Study the drawing (mm; zero at the part's minimum x, y, z) and answer. A direction names the side the tool comes from. Give positions to 0.01 mm unless a question says otherwise; leave off trailing zeros. Write each loop counter-clockwise with the first axis right and the second up, starting at its lowest first coordinate (ties: lowest second). Pieces come first, ordered by that corner, then holes. Notation, with made-up numbers: (32, 74.5) - (44, 74.5) arc R13 ccw to (44, 96.5) - close; hole circle Ø7 at (36, -1). An arc over 180 degrees is marked (long way). Answer as CSV lines item,"result".
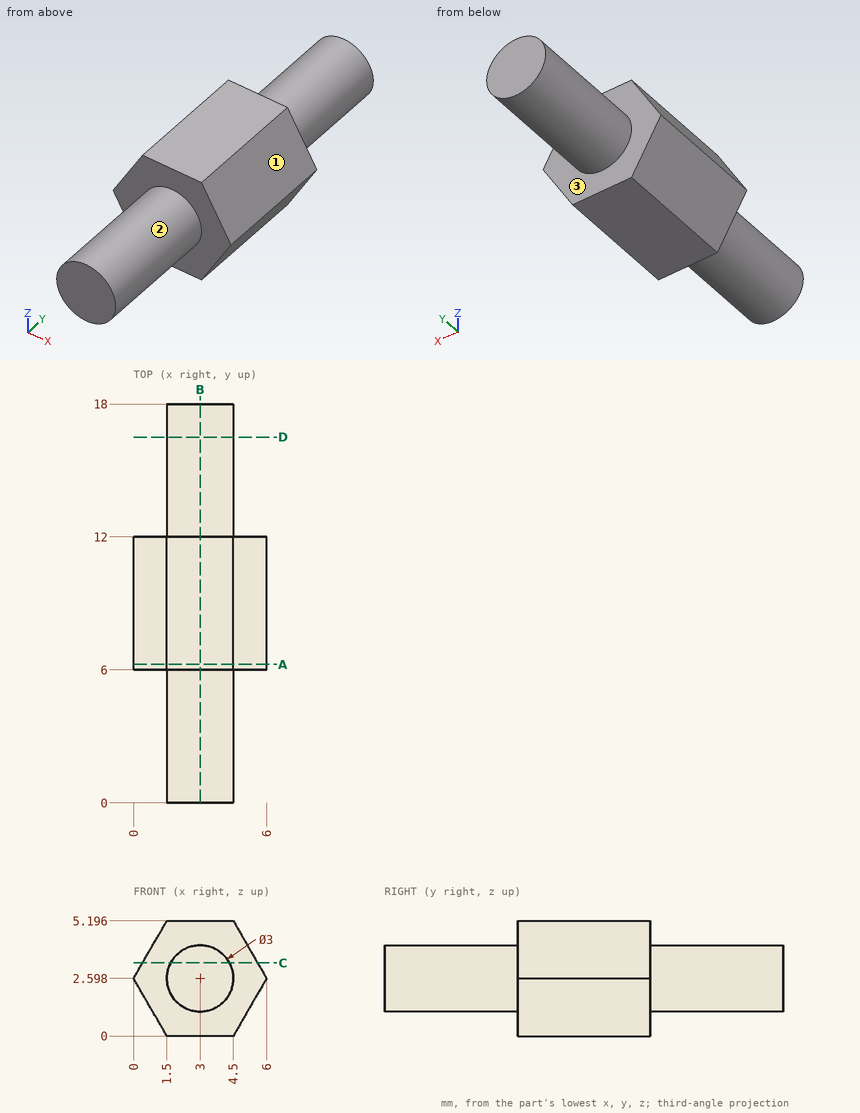
(1) A cutting plane is placed at D-D (y = 16.5). Write down the section's boundary in (x, z).
Worked out:
outline,"circle Ø3 at (3, 2.6)"
(2) Find the intervals of material crossed by L1, parallel to Y at x = 1.6, z = 1.8; L2, parallel to Z at x = 2.9, y = 16.5 (1 decimal); L3, parallel to X at y = 1.5, z = 2.65, in increasing order.
Worked out:
L1,"y = 6 to 12"
L2,"z = 1.1 to 4.1"
L3,"x = 1.5 to 4.5"
(3) For the marked faces 1, 2 and 3, determine the directions among +Z, -Z, +X, -X, +Y, -Y from which every point of the face is accessible in a straight line to the end or side of a thin tool.
Worked out:
face 1,"+Z, +X, +Y, -Y"
face 2,"-Y"
face 3,"+Y"
(4) A cutting plane is placed at B-B (x = 3). Write down the section's boundary in (y, z), and give its area (3 significant figures).
Worked out:
outline,"(0, 1.1) - (6, 1.1) - (6, 0) - (12, 0) - (12, 1.1) - (18, 1.1) - (18, 4.1) - (12, 4.1) - (12, 5.2) - (6, 5.2) - (6, 4.1) - (0, 4.1) - close"
area,"67.2 mm^2"
(5) A cutting plane is placed at A-A (y = 6.25). Write down the section's boundary in (x, z), and give its area (3 significant figures).
Worked out:
outline,"(0, 2.6) - (1.5, 0) - (4.5, 0) - (6, 2.6) - (4.5, 5.2) - (1.5, 5.2) - close"
area,"23.4 mm^2"
(6) A cutting plane is placed at C-C (z = 3.3). Write down the section's boundary in (x, y) (1 decimal).
Worked out:
outline,"(0.4, 6) - (1.7, 6) - (1.7, 0) - (4.3, 0) - (4.3, 6) - (5.6, 6) - (5.6, 12) - (4.3, 12) - (4.3, 18) - (1.7, 18) - (1.7, 12) - (0.4, 12) - close"
(7) Each of these flat-tipped pins is pushed along its axis until it touches: P1, Ø2, axis at y = 10, z = 4.5, coming from the +X side; P2, Ø3, axis at y = 2, z = 1, coming from the +X side. Where does it stop, or does it pass through?
Worked out:
P1,"stops at x = 5.48"
P2,"stops at x = 4.5"
